Geometry: final body of the model. Coordinates: model frame, mm. A direction names the side the tool comes from. Round coordinates to 2 decimals unless told otherwise and drop trailing zeros. Order: outer loops, then holes, each group sorted by start corner. A loop starts at its lowest first (then second) coordinate and runs counter-clockwise, first axis right, second up. Notation, with made-up numbers: M 71.5,-28 L 93.5,-28 A31 ccw 93.5,11 Z; hole C 1.5,-11.5 d1. An arc over 180 degrees is marked long. Return JSON: item names as keys, results as strings. Group by question number.
Q1. Cut plane B-B on z = 2.95. Output: boundary loops of the cut face in (x, y).
Q2. Cut plane A-A on x = 73. Output: boundary loops of the cut face in (y, z), and give its area (3 significant figures).
Q3. Mould query, pull axis X, two halves, no side actions, for faces 3 (the face through (72, 85, 2)), 4 (the face through (0, 49, 2)), 5 (the face through (49, 51, 5)). Classes: released by +X, released by -X, zero draft, split by the parting line, or undercut.
Q4. Access query for faces 1 (the face through (100, 49, 2)), 2 (the face through (35, 17, 2)). Directions: +Z, -Z, +X, -X, +Y, -Y. A direction counts if a zero-diameter tool reaches every point of the face in a straight line with its end or side. Return the directions, or none.
Q5. Ray query, probe 1 along Y at (x, z) = (25, 3.95); probe 2 along Y at (x, z) = (6, 2.1). Return the intervals inside material, ascending.
```python
from build123d import *

# Parameters (mm, degrees)
SKETCH1_W           = 100
SKETCH1_H           = 100
SKETCH1_W_2         = 15
SKETCH1_H_2         = 5
BOSS_EXTRUDE1_DEPTH = 5
FILLET1_R           = 10


with BuildPart() as part:
    # Sketch1 → Boss-Extrude1 (new body)
    with BuildSketch(Plane.XY):
        with Locations((50, 50)):
            Rectangle(SKETCH1_W, SKETCH1_H)
        with Locations((72.5, 82.5)):
            Rectangle(SKETCH1_W_2, SKETCH1_H_2, mode=Mode.SUBTRACT)
        with Locations((27.5, 17.5)):
            Rectangle(SKETCH1_W_2, SKETCH1_H_2, mode=Mode.SUBTRACT)
        with Locations((72.5, 17.5)):
            Rectangle(SKETCH1_W_2, SKETCH1_H_2, mode=Mode.SUBTRACT)
        with Locations((27.5, 82.5)):
            Rectangle(SKETCH1_W_2, SKETCH1_H_2, mode=Mode.SUBTRACT)
    extrude(amount=BOSS_EXTRUDE1_DEPTH)

    # Fillet1
    fillet1_edges = [part.edges().sort_by_distance(p)[0] for p in [
        (0, 100, 2.5),
        (0, 0, 2.5),
    ]]
    fillet(fillet1_edges, radius=FILLET1_R)


solid = part.part
```
Result sheet:
{
 "1": {"outline": "M 0,10 A10 ccw 10,0 L 100,0 L 100,100 L 10,100 A10 ccw 0,90 Z; hole M 20,15 L 35,15 L 35,20 L 20,20 Z; hole M 20,80 L 35,80 L 35,85 L 20,85 Z; hole M 65,15 L 80,15 L 80,20 L 65,20 Z; hole M 65,80 L 80,80 L 80,85 L 65,85 Z"},
 "2": {"outline": "M 0,0 L 15,0 L 15,5 L 0,5 Z; M 20,0 L 80,0 L 80,5 L 20,5 Z; M 85,0 L 100,0 L 100,5 L 85,5 Z", "area": "450 mm²"},
 "3": {"face 3": "undercut", "face 4": "released by -X", "face 5": "zero draft"},
 "4": {"face 1": "+Z, -Z, +X, +Y, -Y", "face 2": "+Z, -Z"},
 "5": {"probe 1": "y = 0 to 15, 20 to 80, 85 to 100", "probe 2": "y = 0.83 to 99.17"}
}
